from build123d import *

# Parameters (mm, degrees)
SKETCH032_W       = 64.5
SKETCH032_H       = 40
PAD013_DEPTH      = 10
SKETCH034_R       = 1.4
PAD014_DEPTH      = 3
SKETCH035_R       = 4
HOLE003_DEPTH     = 18
POCKET015_DEPTH   = 9
POCKET016_DEPTH   = 10.001
SKETCH038_W       = 10
SKETCH038_H       = 10
PAD015_DEPTH      = 15
SKETCH039_R       = 2.5
PAD016_DEPTH      = 5
PAD016_DEPTH_BACK = 15
POCKET017_DEPTH   = 17
POCKET019_DEPTH   = 4


with BuildPart() as part:
    # Sketch032 → Pad013 (new body)
    with BuildSketch(Plane.XZ):
        with Locations((-50.07, -27.33)):
            Rectangle(SKETCH032_W, SKETCH032_H)
    extrude(amount=PAD013_DEPTH)

    # Sketch034 (on Face6 of Pad013) → Pad014 (join)
    with BuildSketch(Plane.XZ.offset(10)):
        with Locations((-79.69, -44.73)):
            Circle(SKETCH034_R)
        with Locations((-79.69, -9.93)):
            Circle(SKETCH034_R)
        with Locations((-30.33, -44.73)):
            Circle(SKETCH034_R)
        with Locations((-30.33, -9.93)):
            Circle(SKETCH034_R)
    extrude(amount=PAD014_DEPTH)

    # Sketch035 (on Face2 of Pad014) → Hole003 (cut)
    with BuildSketch(Plane(origin=(-17.82, 0, 0), x_dir=(0, 0, 1), z_dir=(1, 0, 0))):
        with Locations((-27.33, 5)):
            Circle(SKETCH035_R)
    extrude(amount=-HOLE003_DEPTH, mode=Mode.SUBTRACT)

    # Sketch036 (on Face5 of Hole003) → Pocket015 (cut)
    with BuildSketch(Plane.XZ.offset(10)):
        with BuildLine():
            ThreePointArc((-42.7907317107, -23.1184468896), (-46.935543609, -27.2632587879), (-42.7907317107, -31.4080706862))
            Line((-42.7907317107, -31.4080706862), (-34.7907317107, -31.4080706862))
            ThreePointArc((-34.7907317107, -31.4080706862), (-30.6459198124, -27.2632587879), (-34.7907317107, -23.1184468896))
            Line((-42.7907317107, -23.1184468896), (-34.7907317107, -23.1184468896))
        make_face()
    extrude(amount=-POCKET015_DEPTH, mode=Mode.SUBTRACT)

    # Sketch037 (on Face5 of Pocket015) → Pocket016 (cut, through all)
    with BuildSketch(Plane.XZ.offset(10)):
        Polygon((-8.75606, -47.792807), (-8.75606, -6.792807), (-27.2815885194, -6.792807), (-27.2815885194, -21.225657), (-14.1415885194, -21.225657), (-14.1415885194, -33.274418), (-27.2815885194, -33.274418), (-27.2815885194, -47.792807), align=None)
    extrude(amount=-POCKET016_DEPTH, mode=Mode.SUBTRACT)

    # Sketch038 (on Face7 of Pocket016) → Pad015 (join)
    with BuildSketch(Plane(origin=(-17.82, 0, 0), x_dir=(0, 0, 1), z_dir=(1, 0, 0))):
        with Locations((-27.24382, 5.01)):
            Rectangle(SKETCH038_W, SKETCH038_H)
    extrude(amount=PAD015_DEPTH)

    # Sketch039 (on Face20 of Pad015) → Pad016 (join, two sides)
    with BuildSketch(Plane(origin=(0, 0, -22.24382), x_dir=(-1, 0, 0), z_dir=(0, 0, 1))) as pad016_sk:
        with Locations((7, 5)):
            Circle(SKETCH039_R)
    extrude(amount=PAD016_DEPTH)
    extrude(pad016_sk.sketch, amount=-PAD016_DEPTH_BACK)

    # Sketch040 (on Face31 of Pad016) → Pocket017 (cut)
    with BuildSketch(Plane(origin=(-2.82, 0, 0), x_dir=(0, 0, 1), z_dir=(1, 0, 0))):
        with BuildLine():
            ThreePointArc((-28.743006, 5.2516311207), (-30.6490431207, 3.345594), (-28.743006, 1.4395568793))
            Line((-28.743006, 1.4395568793), (-25.494635, 1.4395568793))
            ThreePointArc((-25.494635, 1.4395568793), (-23.5885978793, 3.345594), (-25.494635, 5.2516311207))
            Line((-28.743006, 5.2516311207), (-25.494635, 5.2516311207))
        make_face()
    extrude(amount=-POCKET017_DEPTH, mode=Mode.SUBTRACT)

    # Sketch045 (on Face21 of Pocket017) → Pocket019 (cut)
    with BuildSketch(Plane(origin=(0, -0.01, 0), x_dir=(1, 0, 0), z_dir=(0, 1, 0))):
        with BuildLine():
            ThreePointArc((-10.990606, 31.0720355), (-14.8442005, 27.218441), (-10.990606, 23.3648465))
            Line((-10.990606, 23.3648465), (5.086273, 23.3648465))
            ThreePointArc((5.086273, 23.3648465), (8.9398675, 27.218441), (5.086273, 31.0720355))
            Line((-10.990606, 31.0720355), (5.086273, 31.0720355))
        make_face()
    extrude(amount=-POCKET019_DEPTH, mode=Mode.SUBTRACT)


with BuildPart() as part_1:
    # Body006 placement: moved
    add(part.part.moved(Location((0, -4, -21))))


solid = part_1.part
Build history of the part. All positions in model axes, mm. A direction names the side the tool comes from. Give positions to 0.01 mm unless a question says otherwise; leave off trailing zeros. Order: outer loops, then holes, each group sorted by start corner. A loop starts at its lowest first (then second) coordinate and runs counter-clockwise, first axis right, second up. Notation, with made-up numbers: M 81,-25.5 L 105,-25.5 A17 ccw 105,-2.5 Z; hole C 61.25,-15.75 d2. An arc over 180 degrees is marked long. Put each result on its own line as item: value.
Item 1: Slice it at C-C, the plane z = -30.93. Write the cut outline in (x, y), plus the area to 3 significant figures.
From the geometry:
outline: M -82.32,-14 L -81.09,-14 L -81.09,-17 L -78.29,-17 L -78.29,-14 L -31.73,-14 L -31.73,-17 L -28.93,-17 L -28.93,-14 L -27.28,-14 L -27.28,-4 L -82.32,-4 Z
area: 567 mm2
Item 2: Slice it at A-A, the plane x = -38. Write the cut outline in (y, z), plus the area to 3 significant figures.
From the geometry:
outline: M -14,-68.33 L -4,-68.33 L -4,-28.33 L -14,-28.33 L -14,-44.12 L -5,-44.12 L -5,-52.41 L -14,-52.41 Z
area: 325 mm2
Item 3: Slice it at D-D, the plane y = -10. Write the cut outline in (x, z), plus the area to 3 significant figures.
From the geometry:
outline: M -82.32,-68.33 L -27.28,-68.33 L -27.28,-54.27 L -17.82,-54.27 L -17.82,-53.24 L -9.29,-53.24 L -9.29,-58.24 L -4.71,-58.24 L -4.71,-53.24 L -2.82,-53.24 L -2.82,-43.24 L -4.71,-43.24 L -4.71,-38.24 L -9.29,-38.24 L -9.29,-43.24 L -17.82,-43.24 L -17.82,-42.23 L -27.28,-42.23 L -27.28,-28.33 L -82.32,-28.33 Z; hole M -42.79,-52.41 L -34.79,-52.41 A4.14 ccw -33.5,-52.2 L -17.82,-52.2 L -17.82,-44.46 L -33.15,-44.46 A4.14 ccw -34.79,-44.12 L -42.79,-44.12 A4.14 ccw Z
area: 2,290 mm2
Item 4: Two-plate mould, pull along Y, no slides. Class faces 6 (the flat face through (-15, -4.01, -48)), 7 (the flat face through (-10, -9.252, -48)), 8 (the cylindrical face through (-30.51, -15.48, -64.34)): +Y half, -Y half, draft (parallel to the pull), parting line (faces both ways), or undercut.
From the geometry:
face 6: +Y half
face 7: undercut
face 8: draft
Item 5: Slice it at B-B, the plane y = -15. Write the cut outline in (x, z), plus the area to 3 significant figures.
From the geometry:
outline: C -79.69,-65.73 d2.8; C -79.69,-30.93 d2.8; C -30.33,-65.73 d2.8; C -30.33,-30.93 d2.8
area: 24.6 mm2
Item 6: Flat gauge pins, fed straight in: pin 1 Ø11 at (x, z) = (-7.5, -50) entering from -Y; pin 2 Ø1.5 at (x, y) = (-6, -9.5) entering from -Z; pin 3 Ø1 at (y, z) = (-9.5, -38) entering from +X. Where does each tip first touch, or does it go through?
From the geometry:
pin 1: stops at y = -14.01
pin 2: stops at z = -58.24
pin 3: stops at x = -4.5
Item 7: Probe line 1 (Y direction, x = -27, z = -48.33); line 2 (X direction, y = -9, z = -56.5); line 3 (Z direction, x = -29.75, y = -9). List the from-to ranges inside material, lowest first. Write a range as [from, to].
From the geometry:
line 1: y = [-14, -13], [-5, -4]
line 2: x = [-82.32, -27.28], [-9.5, -4.5]
line 3: z = [-68.33, -52.33], [-44.33, -28.33]
Item 8: 3-axis set-ups, long thin cutter, end or side, ignore diameter. For faces 1 (the cylindrical face through (-31.36, -15.48, -29.98)), 2 (the flat face through (-2.82, -10, -48)), 3 (the flat face through (-7, -6, -44.365)), 4 (the flat face through (-17.82, -11, -48)), 5 (the flat face through (-22, -9, -54.274)): which of +Z, -Z, +X, -X, +Y, -Y reach the whole face in a straight line?
From the geometry:
face 1: -Y
face 2: +Z, -Z, +X, +Y, -Y
face 3: +X, +Y
face 4: none
face 5: -Z, +Y, -Y
